```python
from build123d import *

# Parameters (mm, degrees)
BOSS_EXTRUDE1_DEPTH   = 180
RIB3_REACH            = 124.404
SKETCH4_WALL_W        = 264.810334732
SKETCH4_WALL_H        = 3
RIB4_START            = -3
RIB4_DEPTH            = 3
F_6_CLEARANCE_HOLE1_D = 3.7973
SKETCH6_R             = 2.3495
CUT_EXTRUDE1_DEPTH    = 7
SKETCH12_R            = 2.6162
CUT_EXTRUDE2_DEPTH    = 6.35
SKETCH13_W            = 5.6
SKETCH13_H            = 180
BOSS_EXTRUDE2_DEPTH   = 5


# Read off the part's stored shape, not the designer's step: Rib4
with BuildPart() as part:
    # Sketch1 → Boss-Extrude1 (new body)
    with BuildSketch(Plane.XY):
        with BuildLine():
            Line((0, 0), (0, 11.25))
            Line((0, 11.25), (-8, 11.25))
            Line((-8, 11.25), (-8, 6))
            ThreePointArc((-8, 6), (-8.878679656, 3.878679656), (-11, 3))
            Line((-11, 3), (-24, 3))
            Line((-24, 3), (-24, 0))
            Line((-24, 0), (0, 0))
        make_face()
    extrude(amount=BOSS_EXTRUDE1_DEPTH)

    # Sketch4 wall → Rib3 (add, up to next)
    with BuildSketch(Plane(origin=(-16, 7.125, 60.5), x_dir=(-0.888803167408, -0.458289133195, 0), z_dir=(-0.458289133195, 0.888803167408, 0)), mode=Mode.PRIVATE) as rib3_sk1:
        Rectangle(SKETCH4_WALL_W, SKETCH4_WALL_H)
    rib3_tool1 = extrude(rib3_sk1.sketch, amount=-RIB3_REACH, mode=Mode.PRIVATE) - part.part
    rib3 = rib3_tool1.solids().sort_by_distance((-16, 7.125, 60.5))[0]
    add(rib3)

    # Rib4 outline → Rib4 (add)
    with BuildSketch(Plane(origin=(0, 0, 0), x_dir=(-1, 0, 0), z_dir=(0, 0, -1)).offset(RIB4_START)):
        with BuildLine():
            Line((24, 3), (8, 11.25))
            Line((8, 11.25), (8, 6))
            ThreePointArc((8, 6), (8.878679656, 3.878679656), (11, 3))
            Line((11, 3), (24, 3))
        make_face()
    rib4 = extrude(amount=RIB4_DEPTH)

    # Mirror1: Rib3, Rib4 across plane
    add(rib3.mirror(Plane(origin=(0, 0, 90), x_dir=(1, 0, 0), z_dir=(0, 0, -1))))
    add(rib4.mirror(Plane(origin=(0, 0, 90), x_dir=(1, 0, 0), z_dir=(0, 0, -1))))

    # #6 Clearance Hole1 (through all)
    with Locations(Plane(origin=(0, 0, 0), x_dir=(-1, 0, 0), z_dir=(0, -1, 0))):
        with Locations((17.5, -31), (17.5, -149), (17.5, -90)):
            Hole(F_6_CLEARANCE_HOLE1_D / 2)

    # Sketch6 → Cut-Extrude1 (cut)
    with BuildSketch(Plane(origin=(0, 0, 0), x_dir=(0, 0, -1), z_dir=(1, 0, 0))):
        with Locations((-149, 5.625)):
            Circle(SKETCH6_R)
        with Locations((-31, 5.625)):
            Circle(SKETCH6_R)
        with Locations((-90, 5.625)):
            Circle(SKETCH6_R)
    extrude(amount=-CUT_EXTRUDE1_DEPTH, mode=Mode.SUBTRACT)

    # Sketch12 → Cut-Extrude2 (cut)
    with BuildSketch(Plane(origin=(0, 0, 0), x_dir=(0, 0, -1), z_dir=(1, 0, 0))):
        with Locations((-149, 5.625)):
            Circle(SKETCH12_R)
        with Locations((-31, 5.625)):
            Circle(SKETCH12_R)
        with Locations((-90, 5.625)):
            Circle(SKETCH12_R)
    extrude(amount=-CUT_EXTRUDE2_DEPTH, mode=Mode.SUBTRACT)

    # Sketch13 → Boss-Extrude2 (add)
    with BuildSketch(Plane(origin=(0, 11.25, 0), x_dir=(1, 0, 0), z_dir=(0, 1, 0))):
        with Locations((-2.8, -90)):
            Rectangle(SKETCH13_W, SKETCH13_H)
    extrude(amount=BOSS_EXTRUDE2_DEPTH)


solid = part.part
```
Source: CAD feature listing. Evaluate the final solid. Frame: model axes, mm. A direction names the side the tool comes from. Give positions to 0.01 mm unless a question says otherwise; leave off trailing zeros. Loops run counter-clockwise (first coordinate to the right, second up) from the corner with the lowest first, then second, coordinate; pieces in that order, holes last. Notation, with made-up numbers: (56, 32) -> (69, 32) arc R27 ccw to (69, 51) -> close; hole circle Ø5 at (71, -20). An arc over 180 degrees is marked (long way). Use a Markdown table: item, result. Add a question column.
(1) Pull-direction query (Y, two-part tool) for faces 4 (the face through (-13, 6, 59)), 5 (the face through (-15.89, 7.18, 60.52)), 6 (the face through (-7, 6, 90)), 7 (the face through (-3.131, 5.74, 33.614)); classes: +Y half, -Y half, draft (parallel to the pull), parting line (faces both ways), or undercut.
(2) First-contact query: pin 1 Ø4 at (y, z) = (5.625, 90) entering from -X; pin 2 Ø6 at (y, z) = (8.5, 97.5) entering from -X; pin 3 Ø1.5 at (x, z) = (-13, 27) entering from +Y. Flat tips, straight axial feed; report the tip coordinate or a pass-through.
(3) Section query A-A (z = 31). Output: boundary loops of the cut face in (x, y).
(4) Section query C-C (y = 13). Output: boundary loops of the cut face in (x, z), then the cut area to 3 significant figures.
(5) Ray query, line 1 (Z direction, x = -17.5, y = 2.15); line 2 (Y direction, x = -2, z = 90); line 3 (X direction, y = 2.3, z = 149). Return the intervals inside material, ascending.
(6) Access query for faces 1 (the face through (-17.747, 1.521, 29.118)), 2 (the face through (-8, 9, 31)), 3 (the face through (-5.6, 14, 91)). Directions: +Z, -Z, +X, -X, +Y, -Y. A direction counts if a zero-diameter tool reaches every point of the face in a straight line with its end or side. Return the directions, or none.
(7) Section query B-B (x = -17.5). Output: boundary loops of the cut face in (y, z), then the cut area to 3 significant figures.
(8) Section query D-D (x = -1.75). Output: boundary loops of the cut face in (y, z) (3 decimals), then the cut area to 3 significant figures.
Checked values:
| question | item | result |
|---|---|---|
| 1 | face 4 | draft |
| 1 | face 5 | +Y half |
| 1 | face 6 | undercut |
| 1 | face 7 | undercut |
| 2 | pin 1 | x = -9.17 |
| 2 | pin 2 | x = -8.04 |
| 2 | pin 3 | y = 3 |
| 3 | outline | (-24, 0) -> (-19.4, 0) -> (-19.4, 3) -> (-24, 3) -> close; (-15.6, 0) -> (0, 0) -> (0, 3.01) -> (-6.35, 3.01) -> (-6.35, 3.28) -> (-7, 3.28) -> (-7, 7.97) -> (-6.35, 7.97) -> (-6.35, 8.24) -> (0, 8.24) -> (0, 16.25) -> (-5.6, 16.25) -> (-5.6, 11.25) -> (-8, 11.25) -> (-8, 6) arc R3 cw to (-11, 3) -> (-15.6, 3) -> close |
| 4 | outline | (-5.6, 0) -> (0, 0) -> (0, 180) -> (-5.6, 180) -> close |
| 4 | area | 1,010 mm^2 |
| 5 | line 1 | 0 to 29.1, 32.9 to 88.1, 91.9 to 147.1, 150.9 to 180 |
| 5 | line 2 | 0 to 3.01, 8.24 to 16.25 |
| 5 | line 3 | -24 to -19.4, -15.6 to 0 |
| 6 | face 1 | +Y, -Y |
| 6 | face 2 | -X, +Y |
| 6 | face 3 | +Z, -Z, -X, +Y |
| 7 | outline | (0, 0) -> (6.35, 0) -> (6.35, 3) -> (3, 3) -> (3, 29.1) -> (0, 29.1) -> close; (0, 32.9) -> (3, 32.9) -> (3, 59) -> (6.35, 59) -> (6.35, 62) -> (3, 62) -> (3, 88.1) -> (0, 88.1) -> close; (0, 91.9) -> (3, 91.9) -> (3, 118) -> (6.35, 118) -> (6.35, 121) -> (3, 121) -> (3, 147.1) -> (0, 147.1) -> close; (0, 150.9) -> (3, 150.9) -> (3, 177) -> (6.35, 177) -> (6.35, 180) -> (0, 180) -> close |
| 7 | area | 546 mm^2 |
| 8 | outline | (0, 0) -> (16.25, 0) -> (16.25, 180) -> (0, 180) -> close; hole circle Ø5.232 at (5.625, 31); hole circle Ø5.232 at (5.625, 90); hole circle Ø5.232 at (5.625, 149) |
| 8 | area | 2,860 mm^2 |
